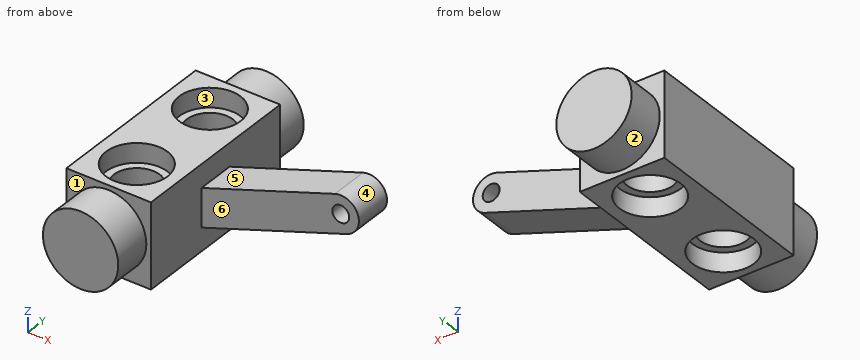
from build123d import *

# Parameters (mm, degrees)
SKETCH1_R           = 4.9
BOSS_EXTRUDE1_DEPTH = 5
SKETCH2_W           = 11
SKETCH2_H           = 11
BOSS_EXTRUDE2_DEPTH = 23
SKETCH3_R           = 4
CUT_EXTRUDE1_DEPTH  = 2.5
SKETCH4_R           = 4
CUT_EXTRUDE2_DEPTH  = 2.5
SKETCH5_R           = 3
CUT_EXTRUDE3_DEPTH  = 6
SKETCH6_R           = 4.9
BOSS_EXTRUDE3_DEPTH = 5
SKETCH7_R           = 1.1
BOSS_EXTRUDE4_DEPTH = 2.5


with BuildPart() as part:
    # Sketch1 → Boss-Extrude1 (new body)
    with BuildSketch(Plane(origin=(0, 0, 0), x_dir=(1, 0, 0), z_dir=(0, 1, 0))):
        Circle(SKETCH1_R)
    extrude(amount=BOSS_EXTRUDE1_DEPTH)

    # Sketch2 → Boss-Extrude2 (add)
    with BuildSketch(Plane(origin=(0, 5, 0), x_dir=(1, 0, 0), z_dir=(0, 1, 0))):
        Rectangle(SKETCH2_W, SKETCH2_H)
    extrude(amount=BOSS_EXTRUDE2_DEPTH)

    # Sketch3 → Cut-Extrude1 (cut)
    with BuildSketch(Plane.XY.offset(5.5)):
        with Locations((0, 10)):
            Circle(SKETCH3_R)
    cut_extrude1 = extrude(amount=-CUT_EXTRUDE1_DEPTH, mode=Mode.SUBTRACT)

    # Sketch4 → Cut-Extrude2 (cut)
    with BuildSketch(Plane(origin=(0, 0, -5.5), x_dir=(-1, 0, 0), z_dir=(0, 0, -1))):
        with Locations((0, 10)):
            Circle(SKETCH4_R)
    cut_extrude2 = extrude(amount=-CUT_EXTRUDE2_DEPTH, mode=Mode.SUBTRACT)

    # Sketch5 → Cut-Extrude3 (cut)
    with BuildSketch(Plane(origin=(0, 0, -3), x_dir=(-1, 0, 0), z_dir=(0, 0, -1))):
        with Locations((0, 10)):
            Circle(SKETCH5_R)
    cut_extrude3 = extrude(amount=-CUT_EXTRUDE3_DEPTH, mode=Mode.SUBTRACT)

    # Sketch6 → Boss-Extrude3 (add)
    with BuildSketch(Plane(origin=(0, 28, 0), x_dir=(1, 0, 0), z_dir=(0, 1, 0))):
        Circle(SKETCH6_R)
    extrude(amount=BOSS_EXTRUDE3_DEPTH)

    # Sketch7 → Boss-Extrude4 (add, symmetric)
    with BuildSketch(Plane(origin=(0, 16.5, 0), x_dir=(1, 0, 0), z_dir=(0, 1, 0))):
        with BuildLine():
            Line((5.5, -2.5), (22.834272834, -8.537145633))
            ThreePointArc((22.834272834, -8.537145633), (25.840339287, -7.084092403), (24.387286057, -4.07802595))
            Line((24.387286057, -4.07802595), (5.5, 2.5))
            Line((5.5, 2.5), (5.5, 0))
            Line((5.5, 0), (5.5, -2.5))
        make_face()
        with Locations((23.610779446, -6.307585792)):
            Circle(SKETCH7_R, mode=Mode.SUBTRACT)
    extrude(amount=BOSS_EXTRUDE4_DEPTH, both=True)

    # Mirror1: Cut-Extrude1 across plane
    add(cut_extrude1.mirror(Plane.ZX.offset(16.5)), mode=Mode.SUBTRACT)

    # Mirror2: Cut-Extrude2 across plane
    add(cut_extrude2.mirror(Plane.ZX.offset(16.5)), mode=Mode.SUBTRACT)

    # Mirror3: Cut-Extrude3 across plane
    add(cut_extrude3.mirror(Plane.ZX.offset(16.5)), mode=Mode.SUBTRACT)


solid = part.part
Check sheet for the modelled part. Datum: model origin and axes. Units: mm. Face numbers are marked on the shaded views. A direction names the side the tool comes from. Round coordinates to 2 decimals unless told otherwise and drop trailing zeros. Loops run counter-clockwise (first coordinate to the right, second up) from the corner with the lowest first, then second, coordinate; pieces in that order, holes last. Notation, with made-up numbers: (68, 3) - (75, 3) arc R23 ccw to (75, 40) - close; hole circle Ø5 at (23, 56.25). An arc over 180 degrees is marked (long way). Answer as CSV lines item,"result". Start each with the question number.
Item 1: Section check C-C (x = 0). Count the separate pieces of the cut face and the enclosed holes in it, and give its area (3 significant figures).
Item 2: Section check A-A (y = 23). Record the boundary of the cut face in (x, z).
Item 3: Depth check by flat-ended pin: P1, Ø2.5, axis at x = 23.61, z = 6.31, coming from the +Y side; P2, Ø12, axis at x = -2.5, y = 19.5, coming from the +Z side; P3, Ø3, axis at y = 23.5, z = -3, coming from the +X side. Enter the tip coordinate at first touch or a pass-through.
Item 4: Scan lines: line 1 (Y direction, x = 0, z = -4.4); line 2 (Y direction, x = 0, z = -0.8); line 3 (X direction, y = 23, z = -1.7). Record each from-to range of solid material in increasing order. Write a range as [from, to].
Item 5: Release check for a two-part mould opening along Z. For the marked faces 4, 5 and 6 record: +Z half, -Z half, draft (parallel to the pull), parting line (faces both ways), or undercut.
Item 6: Section check D-D (y = 13.5). Record the boundary of the cut face in (x, z), and give its area (3 significant figures).
Item 7: Section check B-B (z = -1). Record the boundary of the cut face in (x, y), and give its area (3 significant figures).
Item 8: Set-up check for the marked faces 1, 2 and 3: record each of +Z, -Z, +X, -X, +Y, -Y from which the full face is reachable in a straight line by a thin tool's end or side.
Report:
1,separate pieces,"3"
1,enclosed holes,"0"
1,area,"199 mm2"
2,outline,"(-5.5, -5.5) - (-4, -5.5) - (-4, -3) - (-3, -3) - (-3, 3) - (-4, 3) - (-4, 5.5) - (-5.5, 5.5) - close; (3, -3) - (4, -3) - (4, -5.5) - (5.5, -5.5) - (5.5, 5.5) - (4, 5.5) - (4, 3) - (3, 3) - close"
3,P1,"stops at y = 19"
3,P2,"stops at z = 5.5"
3,P3,"stops at x = 5.5"
4,line 1,"y = [0, 6], [14, 19], [27, 33]"
4,line 2,"y = [0, 7], [13, 20], [26, 33]"
4,line 3,"x = [-5.5, -3], [3, 5.5]"
5,face 4,"parting line"
5,face 5,"+Z half"
5,face 6,"draft"
6,outline,"(-5.5, -5.5) - (-1.94, -5.5) - (-1.94, -3) - (1.94, -3) - (1.94, -5.5) - (5.5, -5.5) - (5.5, 5.5) - (1.94, 5.5) - (1.94, 3) - (-1.94, 3) - (-1.94, 5.5) - (-5.5, 5.5) - close"
6,area,"102 mm2"
7,outline,"(-5.5, 5) - (-4.8, 5) - (-4.8, 0) - (4.8, 0) - (4.8, 5) - (5.5, 5) - (5.5, 14) - (9.81, 14) - (9.81, 19) - (5.5, 19) - (5.5, 28) - (4.8, 28) - (4.8, 33) - (-4.8, 33) - (-4.8, 28) - (-5.5, 28) - close; hole circle Ø6 at (0, 10); hole circle Ø6 at (0, 23)"
7,area,"314 mm2"
8,face 1,"-Y"
8,face 2,"+Y"
8,face 3,"+Z"
